```python
from build123d import *

# Parameters (mm, degrees)
SKETCH1_R           = 2.1
SKETCH1_W           = 42
SKETCH1_H           = 21
BOSS_EXTRUDE1_DEPTH = 10
SKETCH2_W           = 8
SKETCH2_H           = 7.485714894
CUT_EXTRUDE1_DEPTH  = 10
SKETCH3_W           = 7.57739789
SKETCH3_H           = 21
SKETCH3_W_2         = 7.925755829
SKETCH3_H_2         = 20.976807548
CUT_EXTRUDE3_DEPTH  = 3


with BuildPart() as part:
    # Sketch1 → Boss-Extrude1 (new body)
    with BuildSketch(Plane(origin=(0, 0, 0), x_dir=(1, 0, 0), z_dir=(0, 1, 0))):
        with BuildLine():
            Line((-37, 14.15897814), (22, 14.15897814))
            ThreePointArc((22, 14.15897814), (24.444487245, 0.65897814), (22, -12.84102186))
            Line((22, -12.84102186), (-37, -12.84102186))
            ThreePointArc((-37, -12.84102186), (-39.444487245, 0.65897814), (-37, 14.15897814))
        make_face()
        with Locations(Location((15.5, 6.05897814, 0), (0, 0, 270))):
            Circle(SKETCH1_R, mode=Mode.SUBTRACT)
        with Locations(Location((15.5, -3.74102186, 0), (0, 0, 270))):
            Circle(SKETCH1_R, mode=Mode.SUBTRACT)
        with Locations(Location((-33.5, 6.05897814, 0), (0, 0, 90))):
            Circle(SKETCH1_R, mode=Mode.SUBTRACT)
        with Locations(Location((-33.5, -3.74102186, 0), (0, 0, 90))):
            Circle(SKETCH1_R, mode=Mode.SUBTRACT)
        with Locations((-9, 0.65897814)):
            Rectangle(SKETCH1_W, SKETCH1_H, mode=Mode.SUBTRACT)
    extrude(amount=BOSS_EXTRUDE1_DEPTH)

    # Sketch2 → Cut-Extrude1 (cut)
    with BuildSketch(Plane(origin=(0, 0, 0), x_dir=(1, 0, 0), z_dir=(0, 1, 0))):
        with Locations((16, 1.180915362)):
            Rectangle(SKETCH2_W, SKETCH2_H)
    extrude(amount=CUT_EXTRUDE1_DEPTH, mode=Mode.SUBTRACT)

    # Sketch3 → Cut-Extrude3 (cut)
    with BuildSketch(Plane(origin=(0, 0, 0), x_dir=(1, 0, 0), z_dir=(0, 1, 0))):
        with Locations((-33.788698945, 0.65897814)):
            Rectangle(SKETCH3_W, SKETCH3_H)
        with Locations((15.962877914, 0.670574366)):
            Rectangle(SKETCH3_W_2, SKETCH3_H_2)
    extrude(amount=CUT_EXTRUDE3_DEPTH, mode=Mode.SUBTRACT)


solid = part.part
```
For this review, take the finished solid that the model builds, in its own axes (mm). A direction names the side the tool comes from. Coordinates: 2 decimals unless noted, no trailing zeros. Write each loop counter-clockwise with the first axis right and the second up, starting at its lowest first coordinate (ties: lowest second). Pieces come first, ordered by that corner, then holes.
(1) Wall thickness on probe 1 along Z at (x, y) = (-33.5, 5); probe 2 along Z at (x, y) = (-25.5, 5); probe 3 along X at (y, z) = (6.25, -4.75): over which ranges is each line inside the solid? List them lowest first.
(2) For pin 1 Ø1 at (y, z) = (9, 4) entering from +X; pin 2 Ø3 at (x, z) = (-30, -1.5) entering from -Y; pin 3 Ø6 at (y, z) = (5, 6.5) entering from -X, all flat-tipped, find the tip position at first contact; note any pin that passes through.
(3) Tool access review of faces 4 (the face through (-5, 0, 10)), 5 (the face through (12, 6, -8)), 6 (the face through (16, 3, -9)): name each direction out of +Z, -Z, +X, -X, +Y, -Y from which nothing blocks a thin tool from reaching the whole face with its end or side.
(4) Add section A-A on x = -27. Give the boundary of the cut face in (y, z), then the cut area to 3 significant figures.
(5) Add section D-D on z = 4. Give the boundary of the cut face in (x, y), then the cut area to 3 significant figures.
(6) The part is to be moulded in two halves that separate along Z. For faces 1 (the face through (-8, 5, -14.159)), 2 (the face through (-7, 10, -13)), 3 (the face through (-37.577, 1, -1)), say which applies: +Z half, -Z half, draft (parallel to the pull), parting line (faces both ways), or undercut.
(7) Add section B-B on x = -33.5. Give the boundary of the cut face in (y, z).
(8) Add section C-C on y = 5.25. Give the boundary of the cut face in (x, z).
Answer sheet:
1. probe 1: z = -14.16 to -8.16, -3.96 to 1.64, 5.84 to 12.84
1. probe 2: z = -14.16 to -11.16, 9.84 to 12.84
1. probe 3: x = -39.23 to -35.14, -31.86 to -30, 20 to 24.23
2. pin 1: stops at x = 24.22
2. pin 2: stops at y = 3
2. pin 3: stops at x = -39.22
3. face 4: +Z, -Z, +X, -X, -Y
3. face 5: +Y, -Y
3. face 6: -Y
4. outline: (0, -14.16) - (10, -14.16) - (10, -11.16) - (0, -11.16) - close; (0, 9.84) - (10, 9.84) - (10, 12.84) - (0, 12.84) - close
4. area: 60.0 mm2
5. outline: (-39.16, 0) - (-37.58, 0) - (-37.58, 3) - (-35.58, 3) - (-35.58, 10) - (-39.16, 10) - close; (-31.42, 3) - (-30, 3) - (-30, 10) - (-31.42, 10) - close; (12, 3) - (13.42, 3) - (13.42, 10) - (12, 10) - close; (17.58, 3) - (19.93, 3) - (19.93, 0) - (24.16, 0) - (24.16, 10) - (17.58, 10) - close
5. area: 108 mm2
6. face 1: -Z half
6. face 2: draft
6. face 3: undercut
7. outline: (0, -14.16) - (10, -14.16) - (10, -8.16) - (3, -8.16) - (3, -11.16) - (0, -11.16) - close; (0, 9.84) - (3, 9.84) - (3, 5.84) - (10, 5.84) - (10, 12.84) - (0, 12.84) - close; (3, -3.96) - (10, -3.96) - (10, 1.64) - (3, 1.64) - close
8. outline: (-37, -14.16) - (22, -14.16) arc R38.5 ccw to (22, 12.84) - (-37, 12.84) arc R38.5 ccw to start; hole circle Ø4.2 at (-33.5, -6.06); hole circle Ø4.2 at (-33.5, 3.74); hole (-30, -11.16) - (12, -11.16) - (12, -4.92) - (13.73, -4.92) arc R2.1 ccw (long way) to (17.27, -4.92) - (20, -4.92) - (20, 2.56) - (17.24, 2.56) arc R2.1 ccw (long way) to (13.76, 2.56) - (12, 2.56) - (12, 9.84) - (-30, 9.84) - close
